from build123d import *

# Parameters (mm, degrees)
ESQUISSE2_R             = 30
BOSS_EXTRU_1_DEPTH      = 3
ENL_V_MAT_EXTRU_1_DEPTH = 43.532340636
BOSS_EXTRU_3_START      = 6
ESQUISSE5_W             = 10.501413836
ESQUISSE5_H             = 10.144569676
BOSS_EXTRU_3_DEPTH      = 6
ESQUISSE8_R             = 28.75
BOSS_EXTRU_4_DEPTH      = 1.5
BOSS_EXTRU_5_START      = 3
ESQUISSE9_R             = 30
BOSS_EXTRU_5_DEPTH      = 3
ENL_V_MAT_EXTRU_4_DEPTH = 44.370496884
CONG_1_R                = 3
CONG_2_R                = 2
ESQUISSE11_R            = 6.5
AJOURAGE_DEPTH          = 45.522466269


with BuildPart() as part:
    # Esquisse2 → Boss.-Extru.1 (new body)
    with BuildSketch(Plane.XY):
        Circle(ESQUISSE2_R)
    extrude(amount=BOSS_EXTRU_1_DEPTH)

    # Esquisse4 → Enlèv. mat.-Extru.1 (cut, through all)
    with BuildSketch(Plane.XY.offset(3)):
        with BuildLine():
            Line((-2.1, -1.8), (2.1, -1.8))
            ThreePointArc((2.1, -1.8), (2.765863337, 0), (2.1, 1.8))
            Line((2.1, 1.8), (-2.1, 1.8))
            ThreePointArc((-2.1, 1.8), (-2.765863337, 0), (-2.1, -1.8))
        make_face()
    extrude(amount=-ENL_V_MAT_EXTRU_1_DEPTH, mode=Mode.SUBTRACT)

    # Esquisse5 → Boss.-Extru.3 (add)
    with BuildSketch(Plane.XY.offset(3).offset(BOSS_EXTRU_3_START)):
        Rectangle(ESQUISSE5_W, ESQUISSE5_H)
        with BuildLine():
            Line((-2.1, 1.8), (2.1, 1.8))
            ThreePointArc((2.1, 1.8), (2.765863337, 0), (2.1, -1.8))
            Line((2.1, -1.8), (-2.1, -1.8))
            ThreePointArc((-2.1, -1.8), (-2.765863337, 0), (-2.1, 1.8))
        make_face(mode=Mode.SUBTRACT)
    extrude(amount=-BOSS_EXTRU_3_DEPTH)

    # Esquisse8 → Boss.-Extru.4 (add)
    with BuildSketch(Plane(origin=(0, 0, 0), x_dir=(-1, 0, 0), z_dir=(0, 0, -1))):
        Circle(ESQUISSE8_R)
    extrude(amount=BOSS_EXTRU_4_DEPTH)

    # Esquisse9 → Boss.-Extru.5 (add)
    with BuildSketch(Plane(origin=(0, 0, -1.5), x_dir=(-1, 0, 0), z_dir=(0, 0, -1)).offset(BOSS_EXTRU_5_START)):
        with Locations(Location((0, 0, 0), (0, 0, 180))):
            Circle(ESQUISSE9_R)
    extrude(amount=-BOSS_EXTRU_5_DEPTH)

    # Esquisse10 → Enlèv. mat.-Extru.4 (cut, through all)
    with BuildSketch(Plane.XY):
        with BuildLine():
            Line((-2.1, 1.8), (2.1, 1.8))
            ThreePointArc((2.1, 1.8), (2.765863337, 0), (2.1, -1.8))
            Line((2.1, -1.8), (-2.1, -1.8))
            ThreePointArc((-2.1, -1.8), (-2.765863337, 0), (-2.1, 1.8))
        make_face()
    extrude(amount=-ENL_V_MAT_EXTRU_4_DEPTH, mode=Mode.SUBTRACT)

    # Congé1
    # the kernel refuses this fillet: 3 mm, written as the material it takes off along each edge
    with BuildSketch(Plane(origin=(-2.250706918, -2.072284838, 6), x_dir=(-1, 0, 0), z_dir=(0, -1, 0))) as cong_1_piece_1_section:
        Polygon((0, 0), (CONG_1_R, 0), (CONG_1_R, -CONG_1_R), (0, -CONG_1_R), align=None)
    cong_1_piece_1 = extrude(amount=CONG_1_R, mode=Mode.PRIVATE)
    cong_1_piece_1 = cong_1_piece_1 - Plane(origin=(-2.250706918, -2.072284838, 6), x_dir=(0.7071067811865475, 0, -0.7071067811865475), z_dir=(0, -1, 0)) * Sphere(CONG_1_R, mode=Mode.PRIVATE)
    add(cong_1_piece_1, mode=Mode.SUBTRACT)
    with BuildSketch(Plane(origin=(-2.250706918, 2.072284838, 6), x_dir=(-1, 0, 0), z_dir=(0, 1, 0))) as cong_1_piece_2_section:
        Polygon((0, 0), (CONG_1_R, 0), (CONG_1_R, CONG_1_R), (0, CONG_1_R), align=None)
    cong_1_piece_2 = extrude(amount=CONG_1_R, mode=Mode.PRIVATE)
    cong_1_piece_2 = cong_1_piece_2 - Plane(origin=(-2.250706918, 2.072284838, 6), x_dir=(0.7071067811865475, 0, -0.7071067811865475), z_dir=(0, 1, 0)) * Sphere(CONG_1_R, mode=Mode.PRIVATE)
    add(cong_1_piece_2, mode=Mode.SUBTRACT)
    with BuildSketch(Plane(origin=(2.250706918, -2.072284838, 6), x_dir=(0, -1, 0), z_dir=(1, 0, 0))) as cong_1_piece_3_section:
        Polygon((0, 0), (CONG_1_R, 0), (CONG_1_R, -CONG_1_R), (0, -CONG_1_R), align=None)
    cong_1_piece_3 = extrude(amount=CONG_1_R, mode=Mode.PRIVATE)
    cong_1_piece_3 = cong_1_piece_3 - Plane(origin=(2.250706918, -2.072284838, 6), x_dir=(0, 0.7071067811865475, -0.7071067811865475), z_dir=(1, 0, 0)) * Sphere(CONG_1_R, mode=Mode.PRIVATE)
    add(cong_1_piece_3, mode=Mode.SUBTRACT)
    with BuildSketch(Plane(origin=(2.250706918, 2.072284838, 6), x_dir=(1, 0, 0), z_dir=(0, 1, 0))) as cong_1_piece_4_section:
        Polygon((0, 0), (CONG_1_R, 0), (CONG_1_R, -CONG_1_R), (0, -CONG_1_R), align=None)
    cong_1_piece_4 = extrude(amount=CONG_1_R, mode=Mode.PRIVATE)
    cong_1_piece_4 = cong_1_piece_4 - Plane(origin=(2.250706918, 2.072284838, 6), x_dir=(-0.7071067811865475, 0, -0.7071067811865475), z_dir=(0, 1, 0)) * Sphere(CONG_1_R, mode=Mode.PRIVATE)
    add(cong_1_piece_4, mode=Mode.SUBTRACT)
    with BuildSketch(Plane(origin=(-5.250706918, -2.072284838, 9), x_dir=(0, 0, -1), z_dir=(0, 1, 0))) as cong_1_piece_5:
        with BuildLine():
            CenterArc((CONG_1_R, -CONG_1_R), CONG_1_R, 90, 90)
            Line((0, -CONG_1_R), (0, 0))
            Line((0, 0), (CONG_1_R, 0))
        make_face()
    extrude(amount=4.144569676, mode=Mode.SUBTRACT)
    with BuildSketch(Plane(origin=(-5.250706918, 5.072284838, 6), x_dir=(0, -1, 0), z_dir=(0, 0, -1)), Plane(origin=(5.250706918, -5.072284838, 6), x_dir=(0, 1, 0), z_dir=(0, 0, -1)), Plane(origin=(5.250706918, 5.072284838, 6), x_dir=(-1, 0, 0), z_dir=(0, 0, -1))) as cong_1_piece_6:
        with BuildLine():
            CenterArc((CONG_1_R, -CONG_1_R), CONG_1_R, 90, 90)
            Line((0, -CONG_1_R), (0, 0))
            Line((0, 0), (CONG_1_R, 0))
        make_face()
    extrude(amount=3, mode=Mode.SUBTRACT)
    with BuildSketch(Plane(origin=(2.250706918, -5.072284838, 9), x_dir=(0, 1, 0), z_dir=(-1, 0, 0)), Plane(origin=(-2.250706918, 5.072284838, 9), x_dir=(0, -1, 0), z_dir=(1, 0, 0))) as cong_1_piece_7:
        with BuildLine():
            CenterArc((CONG_1_R, CONG_1_R), CONG_1_R, 180, 90)
            Line((0, CONG_1_R), (0, 0))
            Line((0, 0), (CONG_1_R, 0))
        make_face()
    extrude(amount=4.501413836, mode=Mode.SUBTRACT)
    with BuildSketch(Plane(origin=(-5.250706918, -5.072284838, 6), x_dir=(0, 1, 0), z_dir=(0, 0, -1))) as cong_1_piece_8:
        with BuildLine():
            CenterArc((CONG_1_R, CONG_1_R), CONG_1_R, 180, 90)
            Line((0, CONG_1_R), (0, 0))
            Line((0, 0), (CONG_1_R, 0))
        make_face()
    extrude(amount=3, mode=Mode.SUBTRACT)
    with BuildSketch(Plane(origin=(5.250706918, 2.072284838, 9), x_dir=(-1, 0, 0), z_dir=(0, -1, 0))) as cong_1_piece_9:
        with BuildLine():
            CenterArc((CONG_1_R, CONG_1_R), CONG_1_R, 180, 90)
            Line((0, CONG_1_R), (0, 0))
            Line((0, 0), (CONG_1_R, 0))
        make_face()
    extrude(amount=4.144569676, mode=Mode.SUBTRACT)

    # Congé2
    cong_2_edges = [part.edges().sort_by_distance(p)[0] for p in [
        (-5.250706918, 0, 3),
        (0, 5.072284838, 3),
        (0, -5.072284838, 3),
        (5.250706918, 0, 3),
        (-4.372027261, 4.193605182, 3),
        (-4.372027261, -4.193605182, 3),
        (4.372027261, -4.193605182, 3),
        (4.372027261, 4.193605182, 3),
    ]]
    fillet(cong_2_edges, radius=CONG_2_R)

    # Esquisse11 → Ajourage (cut, through all)
    with BuildSketch(Plane(origin=(0, 0, -4.5), x_dir=(-1, 0, 0), z_dir=(0, 0, -1))):
        with Locations((-17, 0)):
            Circle(ESQUISSE11_R)
        with Locations((-5.253288904, 16.167960777)):
            Circle(ESQUISSE11_R)
        with Locations((13.753288904, 9.992349289)):
            Circle(ESQUISSE11_R)
        with Locations((13.753288904, -9.992349289)):
            Circle(ESQUISSE11_R)
        with Locations((-5.253288904, -16.167960777)):
            Circle(ESQUISSE11_R)
    extrude(amount=-AJOURAGE_DEPTH, mode=Mode.SUBTRACT)


solid = part.part
Part model, mm, in its own coordinate system. A direction names the side the tool comes from. Coordinates: 2 decimals unless noted, no trailing zeros. Loops run counter-clockwise (first coordinate to the right, second up) from the corner with the lowest first, then second, coordinate; pieces in that order, holes last. Notation, with made-up numbers: (-12.75, 83.25) - (29.25, 83.25) arc R14 cw to (29.25, 94.25) - close; hole circle Ø4 at (-14, 54.25). An arc over 180 degrees is marked (long way). Write each question's results on one line, items separated by ' | '. Start each with the question number.
Q1. Slice it at A-A on x = 17. Give the cut face in (y, z).
Q2. Slice it at C-C on z = -2.5. Give the cut face in (x, y).
Q3. Which spindle directions (+Z, -Z, +X, -X, +Y, -Y) get a long thin tool onto all of the face, cutting with end or side? Do faces 1 (the cylindrical face through (4.395, -4.17, 5.507)), 2 (the cylindrical face through (4.349, 4.217, 5.507)), 3 (the cylindrical face through (6.232, -28.066, -0.74)), 4 (the cylindrical face through (-2.766, -0.027, 2.344)). Say none if no direction does.
Q4. Slice it at D-D on y = 0. Give the cut face in (x, z), and give its area (3 significant figures).
Q5. Two-plate mould, pull along X, no slides. Class faces 5 (the flat face through (0, -1.8, 2)), 6 (the flat face through (0, 1.8, 2)), 7 (the cylindrical face through (-4.395, -0.029, 8.098)), 8 (the cylindrical face through (0.032, -4.217, 8.098)): +X half, -X half, draft (parallel to the pull), parting line (faces both ways), or undercut.
Q6. Slice it at B-B on y = -18. Give the cut face in (x, z).
Q7. Probe line 1 along Y through (x, z) = (1.5, 0.5); line 2 along Z through (x, y) = (-17, -16); line 3 along X through (y, z) = (-20, -2.75). List the from-to ranges inside material, lowest first.
Q8. Drop flat-ended pins along their axis: pin 1 Ø8 at (y, z) = (11.5, 3.5) entering from -X; pin 2 Ø3 at (y, z) = (-20, -3) entering from +X; pin 3 Ø15 at (x, y) = (-13.75, 9.99) entering from +Z; pin 4 Ø1 at (y, z) = (-7, 4) entering from +X. Give the stop position or say it passes through.
Answer:
1) outline: (-24.72, -4.5) - (-6.5, -4.5) - (-6.5, 3) - (-24.72, 3) - (-24.72, 0) - (-23.19, 0) - (-23.19, -1.5) - (-24.72, -1.5) - close; (6.5, -4.5) - (24.72, -4.5) - (24.72, -1.5) - (23.19, -1.5) - (23.19, 0) - (24.72, 0) - (24.72, 3) - (6.5, 3) - close
2) outline: circle Ø60 at (0, 0); hole circle Ø13 at (-13.75, -9.99); hole circle Ø13 at (-13.75, 9.99); hole (-2.1, -1.8) - (2.1, -1.8) arc R2.77 ccw to (2.1, 1.8) - (-2.1, 1.8) arc R2.77 ccw to start; hole circle Ø13 at (5.25, -16.17); hole circle Ø13 at (5.25, 16.17); hole circle Ø13 at (17, 0)
3) face 1: +Z, +X, -Y | face 2: +Z, +X, +Y | face 3: none | face 4: +Z, -Z
4) outline: (-30, -4.5) - (-2.77, -4.5) - (-2.77, 8.96) arc R3 ccw to (-5.25, 6) - (-5.25, 5) arc R2 cw to (-7.25, 3) - (-30, 3) - (-30, 0) - (-28.75, 0) - (-28.75, -1.5) - (-30, -1.5) - close; (2.77, -4.5) - (10.5, -4.5) - (10.5, 3) - (7.25, 3) arc R2 cw to (5.25, 5) - (5.25, 6) arc R3 ccw to (2.77, 8.96) - close; (23.5, -4.5) - (30, -4.5) - (30, -1.5) - (28.75, -1.5) - (28.75, 0) - (30, 0) - (30, 3) - (23.5, 3) - close | area: 335 mm2
5) face 5: undercut | face 6: undercut | face 7: -X half | face 8: draft
6) outline: (-24, -4.5) - (-0.98, -4.5) - (-0.98, 3) - (-24, 3) - (-24, 0) - (-22.42, 0) - (-22.42, -1.5) - (-24, -1.5) - close; (11.49, -4.5) - (24, -4.5) - (24, -1.5) - (22.42, -1.5) - (22.42, 0) - (24, 0) - (24, 3) - (11.49, 3) - close
7) line 1: y = -29.96 to -21.47, -10.86 to -1.8, 1.8 to 10.86, 21.47 to 29.96 | line 2: z = -4.5 to 3 | line 3: x = -22.36 to 0, 10.5 to 22.36
8) pin 1: stops at x = -29.04 | pin 2: stops at x = 23.62 | pin 3: stops at z = 3 | pin 4: passes through
